Part model, mm, in its own coordinate system. Coordinates: 2 decimals unless noted, no trailing zeros. Write each loop counter-clockwise with the first axis right and the second up, starting at its lowest first coordinate (ties: lowest second). Pieces come first, ordered by that corner, then holes. Notation, with made-up numbers: (-24.75, 63.5) -> (-4.75, 63.5) arc R25 cw to (-4.75, 102.5) -> close; hole circle Ø8 at (-31, -21.5). An arc over 180 degrees is marked (long way). One line per question, with ' | ' between items. Start each with the question number.
Item 1: Saw through at B-B (x = 67.5). List the corners of the cut face in (y, z), and give its area (3 significant figures).
Item 2: Saw through at A-A (z = -15). List the corners of the cut face in (x, y) (3 decimals), and give its area (3 significant figures).
Item 3: Pin check, flat tips, straight feed: pin 1 (7 mm diameter, centred on x = -14.375, z = 15, fed in from -Y); pin 2 (5.5 mm diameter, centred on x = 67.5, z = -47.5, fed in from -Y). Stop position of each tip, or through.
Item 4: Probe probe 1 along X at (y, z) = (3, -22.25); probe 2 along X at (y, z) = (1.5, 47.5); probe 3 along X at (y, z) = (4.5, 15) (3 decimals). List the from-to ranges inside material, lowest first. Write a range as [from, to].
Item 5: Two-plate mould, pull along Z, no slides. Class faces 1 (the cylindrical face through (79.61, 3.131, -19.752)), 2 (the flat face through (-110, 3, 1)): pulls with the +Z half, pulls with the -Z half, needs draft (parallel to the pull), parting line crosses it, or undercut.
Item 6: Saw through at C-C (x = -79.5). List the corners of the cut face in (y, z).
Item 7: Saw through at D-D (y = 2.75). Count the separate pieces of the cut face and the enclosed holes in it, and give its area (3 significant figures).
from build123d import *

# Parameters (mm, degrees)
SKETCH1_W                 = 200
SKETCH1_H                 = 110
BOSS_EXTRUDE1_DEPTH       = 6.35
M6_CLEARANCE_HOLE1_D      = 6.6
M6_CLEARANCE_HOLE1_DEPTH  = 12.4
M6_CLEARANCE_HOLE1_TIP    = 1.982840043
EXTENDO_W                 = 10
EXTENDO_H                 = 110
BOSS_EXTRUDE2_DEPTH       = 6.35
M6X1_0_TAPPED_HOLE2_D     = 5
M6X1_0_TAPPED_HOLE2_DEPTH = 15
M6X1_0_TAPPED_HOLE2_TIP   = 1.502151548
M4_CLEARANCE_HOLE2_D      = 4.5
M4_CLEARANCE_HOLE2_DEPTH  = 15
M4_CLEARANCE_HOLE2_TIP    = 1.351936393
M4_CLEARANCE_HOLE3_D      = 4.5
M4_CLEARANCE_HOLE3_DEPTH  = 15
M4_CLEARANCE_HOLE3_TIP    = 1.351936393
SKETCH20_W                = 12.5
SKETCH20_H                = 110
CUT_EXTRUDE1_DEPTH        = 6.35


with BuildPart() as part:
    # Sketch1 → Boss-Extrude1 (new body)
    with BuildSketch(Plane(origin=(0, 0, 0), x_dir=(1, 0, 0), z_dir=(0, 1, 0))):
        Rectangle(SKETCH1_W, SKETCH1_H)
    extrude(amount=BOSS_EXTRUDE1_DEPTH)

    # M6 Clearance Hole1
    with Locations(Plane(origin=(-67.5, 6.35, -47.5), x_dir=(0, 0, 1), z_dir=(0, 1, 0))):
        with Locations((0, 0), (0, 40), (40, 40), (40, 0), (55, 0), (55, 40), (95, 40), (95, 0), (95, 95), (55, 95), (40, 95), (0, 95), (0, 135), (40, 135), (55, 135), (95, 135)):
            Hole(M6_CLEARANCE_HOLE1_D / 2, depth=M6_CLEARANCE_HOLE1_DEPTH)
            with Locations((0, 0, -(M6_CLEARANCE_HOLE1_DEPTH + M6_CLEARANCE_HOLE1_TIP / 2))):  # 118° drill point
                Cone(0, M6_CLEARANCE_HOLE1_D / 2, M6_CLEARANCE_HOLE1_TIP, mode=Mode.SUBTRACT)

    # Extendo → Boss-Extrude2 (add)
    with BuildSketch(Plane(origin=(0, 6.35, 0), x_dir=(1, 0, 0), z_dir=(0, 1, 0))):
        with Locations((-105, 0)):
            Rectangle(EXTENDO_W, EXTENDO_H)
    extrude(amount=-BOSS_EXTRUDE2_DEPTH)

    # M6x1.0 Tapped Hole2
    with Locations(Plane(origin=(-79.5, 6.35, -22.25), x_dir=(0, 0, 1), z_dir=(0, 1, 0))):
        with Locations((0, 0), (44.5, 0), (44.5, 159), (0, 159)):
            Hole(M6X1_0_TAPPED_HOLE2_D / 2, depth=M6X1_0_TAPPED_HOLE2_DEPTH)
            with Locations((0, 0, -(M6X1_0_TAPPED_HOLE2_DEPTH + M6X1_0_TAPPED_HOLE2_TIP / 2))):  # 118° drill point
                Cone(0, M6X1_0_TAPPED_HOLE2_D / 2, M6X1_0_TAPPED_HOLE2_TIP, mode=Mode.SUBTRACT)

    # M4 Clearance Hole2
    with Locations(Plane(origin=(-104.5, 6.35, -22.25), x_dir=(0, 0, 1), z_dir=(0, 1, 0))):
        with Locations((0, 0), (44.5, 0)):
            Hole(M4_CLEARANCE_HOLE2_D / 2, depth=M4_CLEARANCE_HOLE2_DEPTH)
            with Locations((0, 0, -(M4_CLEARANCE_HOLE2_DEPTH + M4_CLEARANCE_HOLE2_TIP / 2))):  # 118° drill point
                Cone(0, M4_CLEARANCE_HOLE2_D / 2, M4_CLEARANCE_HOLE2_TIP, mode=Mode.SUBTRACT)

    # M4 Clearance Hole3
    with Locations(Plane(origin=(-14.375, 6.35, -15), x_dir=(0, 0, 1), z_dir=(0, 1, 0))):
        with Locations((0, 0), (30, 0)):
            Hole(M4_CLEARANCE_HOLE3_D / 2, depth=M4_CLEARANCE_HOLE3_DEPTH)
            with Locations((0, 0, -(M4_CLEARANCE_HOLE3_DEPTH + M4_CLEARANCE_HOLE3_TIP / 2))):  # 118° drill point
                Cone(0, M4_CLEARANCE_HOLE3_D / 2, M4_CLEARANCE_HOLE3_TIP, mode=Mode.SUBTRACT)

    # Sketch20 → Cut-Extrude1 (cut)
    with BuildSketch(Plane(origin=(0, 6.35, 0), x_dir=(1, 0, 0), z_dir=(0, 1, 0))):
        with Locations((93.75, 0)):
            Rectangle(SKETCH20_W, SKETCH20_H)
    extrude(amount=-CUT_EXTRUDE1_DEPTH, mode=Mode.SUBTRACT)


solid = part.part
From the geometry:
1) outline: (0, -55) -> (6.35, -55) -> (6.35, -50.8) -> (0, -50.8) -> close; (0, -44.2) -> (6.35, -44.2) -> (6.35, -10.8) -> (0, -10.8) -> close; (0, -4.2) -> (6.35, -4.2) -> (6.35, 4.2) -> (0, 4.2) -> close; (0, 10.8) -> (6.35, 10.8) -> (6.35, 44.2) -> (0, 44.2) -> close; (0, 50.8) -> (6.35, 50.8) -> (6.35, 55) -> (0, 55) -> close | area: 531 mm2
2) outline: (-110, 0) -> (-16.625, 0) -> (-16.625, 6.35) -> (-110, 6.35) -> close; (-12.125, 0) -> (87.5, 0) -> (87.5, 6.35) -> (-12.125, 6.35) -> close | area: 1,230 mm2
3) pin 1: y = 0 | pin 2: through
4) probe 1: [-110, -106.75], [-102.25, -82], [-77, 77], [82, 87.5] | probe 2: [-110, -70.8], [-64.2, -30.8], [-24.2, 24.2], [30.8, 64.2], [70.8, 87.5] | probe 3: [-110, -16.625], [-12.125, 87.5]
5) face 1: undercut | face 2: needs draft
6) outline: (0, -55) -> (6.35, -55) -> (6.35, -24.75) -> (0, -24.75) -> close; (0, -19.75) -> (6.35, -19.75) -> (6.35, 19.75) -> (0, 19.75) -> close; (0, 24.75) -> (6.35, 24.75) -> (6.35, 55) -> (0, 55) -> close
7) separate pieces: 1 | enclosed holes: 24 | area: 21,000 mm2
